from build123d import *

# Parameters (mm, degrees)
SKETCH1_W                = 25
SKETCH1_H                = 38
SKETCH1_W_2              = 16.5
SKETCH1_H_2              = 1.4
BOSS_EXTRUDE1_DEPTH      = 2
SKETCH1_3_W              = 16.5
SKETCH1_3_H              = 1.4
BOSS_EXTRUDE2_DEPTH      = 5.5
BOSS_EXTRUDE3_DEPTH      = 3
BOSS_EXTRUDE3_DEPTH_BACK = 3
SKETCH3_W                = 6.5
SKETCH3_H                = 1.4
CUT_EXTRUDE1_DEPTH       = 3.5


with BuildPart() as part:
    # Sketch1 → Boss-Extrude1 (new body)
    with BuildSketch(Plane(origin=(0, 0, 0), x_dir=(1, 0, 0), z_dir=(0, 1, 0))):
        Rectangle(SKETCH1_W, SKETCH1_H)
        with Locations((0, -17.2)):
            Rectangle(SKETCH1_W_2, SKETCH1_H_2, mode=Mode.SUBTRACT)
        with Locations((0, 17.2)):
            Rectangle(SKETCH1_W_2, SKETCH1_H_2, mode=Mode.SUBTRACT)
    extrude(amount=BOSS_EXTRUDE1_DEPTH)

    # Sketch1<3> → Boss-Extrude2 (add)
    with BuildSketch(Plane(origin=(0, 0, 0), x_dir=(1, 0, 0), z_dir=(0, 1, 0))):
        Polygon((-14, -1.5), (-12.5, -3), (-12.5, 3), (-14, 1.5), align=None)
        Polygon((12.5, 3), (12.5, -3), (14, -1.5), (14, 1.5), align=None)
        with Locations((0, 17.2)):
            Rectangle(SKETCH1_3_W, SKETCH1_3_H)
        with Locations((0, -17.2)):
            Rectangle(SKETCH1_3_W, SKETCH1_3_H)
    extrude(amount=BOSS_EXTRUDE2_DEPTH)

    # Sketch2 → Boss-Extrude3 (add, two sides: drawn at the far end of the back side and taken through both)
    with BuildSketch(Plane.XY.offset(-BOSS_EXTRUDE3_DEPTH_BACK)):
        Polygon((12.5, 5.5), (11.5, 4.5), (12.5, 4.5), align=None)
        Polygon((-11.5, 4.5), (-12.5, 4.5), (-12.5, 5.5), align=None)
    extrude(amount=BOSS_EXTRUDE3_DEPTH + BOSS_EXTRUDE3_DEPTH_BACK)

    # Sketch3 → Cut-Extrude1 (cut)
    with BuildSketch(Plane(origin=(0, 2, 0), x_dir=(1, 0, 0), z_dir=(0, 1, 0))):
        with Locations((0, -17.2)):
            Rectangle(SKETCH3_W, SKETCH3_H)
    extrude(amount=CUT_EXTRUDE1_DEPTH, mode=Mode.SUBTRACT)


solid = part.part
Input: part model. Units: mm. Frame: model coordinates. A direction names the side the tool comes from. Give positions to 0.01 mm unless a question says otherwise; leave off trailing zeros. Write each loop counter-clockwise with the first axis right and the second up, starting at its lowest first coordinate (ties: lowest second). Pieces come first, ordered by that corner, then holes.
Q1. Section D-D, the plane y = 1.25. Output: boundary loops of the cut face in (x, z), plus the area to 4 significant figures.
Q2. Pull-direction query (X, two-part tool) for faces 6 (the face through (-14, 3, 0)), 7 (the face through (12, 5, 0)), 8 (the face through (-12.2, 4.8, 3)); classes: pulls with the +X half, pulls with the -X half, needs draft (parallel to the pull), parting line crosses it, or undercut.
Q3. Section B-B, the plane x = -0.5. Output: boundary loops of the cut face in (y, z), plus the area to 3 significant figures.
Q4. Section C-C, the plane z = 0. Output: boundary loops of the cut face in (x, y), plus the area to 3 significant figures.
Q5. First-contact query: P1, Ø0.7, axis at y = 4, z = 17, coming from the -X side; P2, Ø1, axis at y = 1, z = -12, coming from the -X side; P3, Ø3, axis at x = -6, y = 4, coming from the -Z side. Flat tips, straight axial feed; report the tip coordinate or a pass-through.
Q6. Set-up query: faces 1 (the face through (-6, 4, 17.9)), 2 (the face through (12.5, 3, 0)), 3 (the face through (6, 4, 16.5)), 4 (the face through (-12, 5, 0)), 5 (the face through (0, 4, -17.9)). Return all of +Z, -Z, +X, -X, +Y, -Y with unobstructed straight access to the full face (end or side cutting, diameter ignored); none if empty.
Q7. Material intervals for probe 1 along Z at (x, y) = (4.25, 3.7); probe 2 along X at (y, z) = (0.25, 12.5); probe 3 along Y at (x, z) = (-0.5, -11.5), sorted ascending.
Q8. Section A-A, the plane y = 5. Output: boundary loops of the cut face in (x, z).
Filled in:
1. outline: (-14, -1.5) - (-12.5, -3) - (-12.5, -19) - (12.5, -19) - (12.5, -3) - (14, -1.5) - (14, 1.5) - (12.5, 3) - (12.5, 19) - (-12.5, 19) - (-12.5, 3) - (-14, 1.5) - close
1. area: 963.5 mm2
2. face 6: pulls with the -X half
2. face 7: undercut
2. face 8: needs draft
3. outline: (0, -19) - (2, -19) - (2, -17.9) - (5.5, -17.9) - (5.5, -16.5) - (2, -16.5) - (2, 19) - (0, 19) - close
3. area: 80.9 mm2
4. outline: (-14, 0) - (14, 0) - (14, 5.5) - (12.5, 5.5) - (11.5, 4.5) - (12.5, 4.5) - (12.5, 2) - (-12.5, 2) - (-12.5, 4.5) - (-11.5, 4.5) - (-12.5, 5.5) - (-14, 5.5) - close
4. area: 67.5 mm2
5. P1: stops at x = -8.25
5. P2: stops at x = -12.5
5. P3: stops at z = -17.9
6. face 1: +Z, +X, -X, +Y
6. face 2: +Z, -Z
6. face 3: +X, -X, +Y
6. face 4: +Z, -Z, +Y
6. face 5: -Z, +X, -X, +Y
7. probe 1: z = -17.9 to -16.5, 16.5 to 17.9
7. probe 2: x = -12.5 to 12.5
7. probe 3: y = 0 to 2
8. outline: (-14, -1.5) - (-12.5, -3) - (-12, -3) - (-12, 3) - (-12.5, 3) - (-14, 1.5) - close; (-8.25, -17.9) - (8.25, -17.9) - (8.25, -16.5) - (-8.25, -16.5) - close; (-8.25, 16.5) - (-3.25, 16.5) - (-3.25, 17.9) - (-8.25, 17.9) - close; (3.25, 16.5) - (8.25, 16.5) - (8.25, 17.9) - (3.25, 17.9) - close; (12, -3) - (12.5, -3) - (14, -1.5) - (14, 1.5) - (12.5, 3) - (12, 3) - close
